Geometry check sheet. Reference: the model listing, model coordinates, mm. Face numbers are marked on the shaded views. A direction names the side the tool comes from. Give positions to 0.01 mm unless a question says otherwise; leave off trailing zeros. Loops run counter-clockwise (first coordinate to the right, second up) from the corner with the lowest first, then second, coordinate; pieces in that order, holes last. Notation, with made-up numbers: (-38, -4) - (-7, -4) arc R22 ccw to (-7, 30) - close; hole circle Ø4 at (29.25, 79.25). An arc over 180 degrees is marked (long way). Use a Markdown table: item, result. Add a question column.
1. Cross-section at B-B on x = -517. Enter the section's corners in (y, z).
2. Material ranges on L1, parallel to X at y = 2.25, z = -630; L2, parallel to Z at x = -517, y = 2.05; L3, parallel to Y at x = -513, z = -506, recorded low to high.
3. Depth check by flat-ended pin: P1, Ø3.5, axis at x = -371, y = 2, coming from the -Z side; P2, Ø10, axis at y = 19, z = -523.5, coming from the +X side; P3, Ø0.9, axis at y = 1.5, z = -613.5, coming from the +X side. Enter the tip coordinate at first touch or a pass-through.
4. Set-up check for the marked faces 1 and 2: record each of +Z, -Z, +X, -X, +Y, -Y from which the full face is reachable in a straight line by a thin tool's end or side.
5. Cross-section at A-A on z = -630. Enter the section's corners in (x, y).
6. Cross-section at C-C on z = -552. Enter the section's corners in (x, y), and give its area (3 significant figures).
7. Cross-section at D-D on y = 11. Enter the section's corners in (x, z), and give its area (3 significant figures).
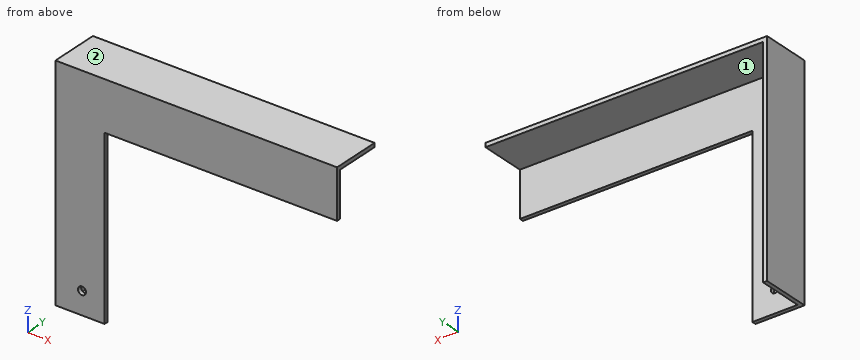
Autodesk Inventor part; units mm, degrees
ref_plane "YZ Plane" through (0, 0, 0) normal (1, 0, 0) x (0, 1, 0)
ref_plane "XZ Plane" through (0, 0, 0) normal (0, 1, 0) x (-1, 0, 0)
ref_plane "XY Plane" through (0, 0, 0) normal (0, 0, 1) x (1, 0, 0)
sketch "Sketch1" plane through (0, 0, 0) normal (0, 1, 0) x (-1, 0, 0)
  line L0 (0, 0) -> (0, -650)
  line L1 (0, -650) -> (650, -650)
  line L2 (650, -650) -> (650, 0)
  line L3 (650, 0) -> (0, 0)
  line L4 (0, 0) -> (3, 0)
  line L5 (3, -3) -> (3, -647)
  line L6 (3, -650) -> (0, -650)
  line L7 (0, -650) -> (0, -647)
  line L8 (650, -647) -> (650, -650)
  line L9 (650, -650) -> (647, -650)
  line L10 (647, -650) -> (647, 0)
  line L11 (647, 0) -> (650, 0)
  line L12 (650, 0) -> (650, -3)
  line L13 (0, -3) -> (0, 0)
  line L14 (0, 0) -> (0, -37)
  line L15 (650, -37) -> (650, 0)
  line L16 (650, 0) -> (613, 0)
  line L17 (613, 0) -> (613, -650)
  line L18 (613, -650) -> (650, -650)
  line L19 (650, -650) -> (650, -613)
  line L20 (0, -613) -> (0, -650)
  line L21 (0, -650) -> (37, -650)
  line L22 (37, 0) -> (0, 0)
  line L23 (3, -147.3087) -> (3, -94.9828)
  line L24 (147.3087, -3) -> (94.9828, -3)
  circle A0 centre (16.1109, -108.0348) radius 3
  line L25 (0, -650) -> (3, -650)
  line L26 (0, -647) -> (0, -650)
  line L27 (0, -650) -> (0, -613)
  line L28 (37, -650) -> (0, -650)
  line L29 (3, -502.6913) -> (3, -555.0172)
  line L30 (147.3087, -647) -> (94.9828, -647)
  circle A1 centre (16.1109, -541.9652) radius 3
  line L31 (37, -650) -> (37, -37)
  line L32 (37, -3) -> (37, 0)
  line L33 (650, -3) -> (34.9546, -3)
  line L34 (34.9546, -647) -> (650, -647)
  line L35 (37, -37) -> (0, 0)
  line L36 (37, -613) -> (0, -650)
  line L37 (0, -650) -> (3, -647)
  line L38 (3, -647) -> (3, -3)
  line L39 (3, -3) -> (0, 0)
  line L40 (3, -325) -> (3, -458)
  line L41 (3, -458) -> (20, -458)
  line L42 (3, -325) -> (3, -192)
  line L43 (3, -192) -> (20, -192)
  circle A2 centre (20, -192) radius 3
  circle A3 centre (20, -458) radius 3
  line L44 (325, -650) -> (192, -650)
  circle A4 centre (192, -630) radius 3
  line L45 (3, -458) -> (3, -475)
  line L46 (3, -475) -> (647, -475)
  line L47 (3, -475) -> (3, -478)
  line L48 (3, -478) -> (647, -478)
  line L49 (175, -630) -> (175, -481)
  line L50 (175, -630) -> (175, -647)
  line L51 (209, -630) -> (209, -647)
  line L52 (209, -647) -> (175, -647)
  line L53 (175, -647) -> (172, -647)
  line L54 (172, -647) -> (172, -478)
  line L55 (325, -650) -> (325, -478)
  line L56 (325, -478) -> (172, -478)
  line L57 (325, -481) -> (175, -481)
  line L58 (325, -515) -> (209, -515)
  line L59 (209, -630) -> (209, -515)
  line L60 (650, -650) -> (517, -650)
  line L61 (517, -650) -> (517, -647)
  line L62 (517, -647) -> (517, -630)
  line L63 (517, -647) -> (500, -647)
  line L64 (517, -647) -> (534, -647)
  circle A5 centre (517, -630) radius 3
  line L65 (534, -647) -> (534, -481)
  line L66 (325, -478) -> (325, -515)
  line L67 (325, -515) -> (500, -515)
  line L68 (534, -481) -> (325, -481)
  line L69 (325, -481) -> (325, -478)
  line L70 (500, -647) -> (500, -515)
  line L71 (534, -478) -> (537, -478)
  line L72 (537, -478) -> (537, -647)
  line L73 (537, -647) -> (534, -647)
  point P0 (37, -647)
  dimension "d0" = 650
  dimension "d1" = 650
  dimension "d2" = 650
  dimension "d3" = 3
  dimension "d4" = 650
  dimension "d5" = 3
  dimension "d6" = 3
  dimension "d7" = 650
  dimension "d8" = 3
  dimension "d9" = 650
  dimension "d10" = 37
  dimension "d12" = 37
  dimension "d13" = 650
  dimension "d14" = 37
  dimension "d15" = 650
  dimension "d16" = 37
  dimension "d28" = 6
  dimension "d33" = 133
  dimension "d34" = 17
  dimension "d35" = 133
  dimension "d36" = 17
  dimension "d37" = 6
  dimension "d38" = 6
  dimension "d41" = 133
  dimension "d43" = 6
  dimension "d44" = 17
  dimension "d45" = 3
  dimension "d47" = 17
  dimension "d48" = 3
  dimension "d55" = 133
  dimension "d56" = 17
  dimension "d57" = 17
  dimension "d58" = 17
  dimension "d59" = 6
  dimension "d60" = 37
  dimension "d61" = 3
  dimension "d62" = 3
extrude "Extrusion6" add sketch "Sketch1" along normal blind 3 contours L68 L65 L34 L70 L67 L55
extrude "Extrusion7" add sketch "Sketch1" along normal blind 37 contours L48 L72 L34 L65 L68 L55
properties part number "body_inner_L_support(2)"
Values found:
| question | item | result |
|---|---|---|
| 1 | outline | (0, -647) - (3, -647) - (3, -633) - (0, -633) - close; (0, -627) - (3, -627) - (3, -481) - (37, -481) - (37, -478) - (0, -478) - close |
| 2 | L1 | x = -537 to -520, -514 to -500 |
| 2 | L2 | z = -647 to -633, -627 to -478 |
| 2 | L3 | y = 0 to 3 |
| 3 | P1 | stops at z = -515 |
| 3 | P2 | stops at x = -534 |
| 3 | P3 | stops at x = -500 |
| 4 | face 1 | -Z, +X, +Y |
| 4 | face 2 | +Z, +X, -X, +Y, -Y |
| 5 | outline | (-537, 0) - (-520, 0) - (-520, 3) - (-534, 3) - (-534, 37) - (-537, 37) - close; (-514, 0) - (-500, 0) - (-500, 3) - (-514, 3) - close |
| 6 | outline | (-537, 0) - (-500, 0) - (-500, 3) - (-534, 3) - (-534, 37) - (-537, 37) - close |
| 6 | area | 213 mm2 |
| 7 | outline | (-537, -647) - (-534, -647) - (-534, -481) - (-325, -481) - (-325, -478) - (-537, -478) - close |
| 7 | area | 1,130 mm2 |
